from build123d import *

# Parameters (mm, degrees)
F0_W     = 60.325
F0_H     = 104.775
F1_DEPTH = 66.675
F3_DEPTH = 34.925
F5_DEPTH = 22.225
F6_W     = 26.9875
F6_H     = 6.35
F6_W_2   = 25.4
F7_DEPTH = 60.326
F9_DEPTH = 60.326


with BuildPart() as f1:
    # F0 (on Top) → F1 (new body)
    with BuildSketch(Plane.XY):
        Rectangle(F0_W, F0_H)
    extrude(amount=F1_DEPTH)

    # F2 (on face) → F3 (cut)
    with BuildSketch(Plane.YZ.offset(30.1625)):
        Polygon((-52.3875, 34.8233953258), (-52.3875, 15.875), (52.3875, 41.275), (52.3875, 60.2233953258), align=None)
    extrude(amount=-F3_DEPTH, mode=Mode.SUBTRACT)

    # F4 (on face) → F5 (cut)
    with BuildSketch(Plane.YZ.offset(30.1625)):
        Polygon((7.9375, 0), (7.9375, 30.4992424242), (-26.9875, 22.0325757576), (-26.9875, 0), align=None)
    extrude(amount=-F5_DEPTH, mode=Mode.SUBTRACT)

    # F6 (on face) → F7 (cut, through all)
    with BuildSketch(Plane.YZ.offset(30.1625)):
        with Locations((-13.49375, 3.175)):
            Rectangle(F6_W, F6_H)
        with Locations((-39.6875, 3.175)):
            Rectangle(F6_W_2, F6_H)
        Polygon((52.8014078736, 0), (52.5065548718, 6.35), (20.6375, 6.35), (20.6375, 0), align=None)
    extrude(amount=-F7_DEPTH, mode=Mode.SUBTRACT)

    # F8 (on face) → F9 (cut, through all)
    with BuildSketch(Plane.YZ.offset(30.1625)):
        Polygon((-7.9375, 45.5991529015), (-7.9375, 66.675), (-52.3875, 66.675), (-52.3875, 34.8233953258), align=None)
    extrude(amount=-F9_DEPTH, mode=Mode.SUBTRACT)


solid = f1.part
Can you work these out from the model? Positions are in its coordinate system, mm. A direction names the side the tool comes from. Coordinates: 2 decimals unless noted, no trailing zeros. Loops run counter-clockwise (first coordinate to the right, second up) from the corner with the lowest first, then second, coordinate; pieces in that order, holes last. Notation, with made-up numbers: M 1.5,28.5 L 7.5,28.5 A24 cw 7.5,39.5 Z; hole C -30,86 d4. An arc over 180 degrees is marked long. Return JSON: item names as keys, results as strings. Group by question number.
Item 1: Imagine slicing it at A-A (x = 22.5). Give the number of separate pieces and of enclosed holes in the cut face, and give its area (3 significant figures).
Item 2: On a 3-axis mill with a long thin cutter (end or side, diameter ignored), from which of +Z, -Z, +X, -X, +Y, -Y can I reach the whole of each face in a straight line? I mean faces 5 (the flat face through (0, 20.638, 3)), 6 (the flat face through (-6, -26, 6.35)), 7 (the flat face through (19, -26.988, 14)), 8 (the flat face through (7.938, -6, 15)). Say none if no direction works.
Item 3: I'm going to push flat-ended pins straight in: pin 1 Ø1.9 at (x, z) = (-19.5, 2.5) entering from -Y; pin 2 Ø3 at (x, z) = (5.5, 2) entering from +Y; pin 3 Ø1 at (x, z) = (-1.5, 56.5) entering from -Y; pin 4 Ø5 at (x, y) = (12, -22.5) entering from -Z. Where does each tip first touch, or does it pass through?
Item 4: Imagine slicing it at C-C (z = 13.5). Please give me the cut outline in (x, y).
Item 5: If I drill on L1, parallel to Z at x = -14, y = 29 (3 decimals); L2, parallel to Z at x = -4, y = 48 (3 decimals); L3, parallel to Y at x = -13, z = 3, over which ranges is the centre line in solid material (lowest first)? Write a range as from..to.
Item 6: Thinking about a two-plate mould opening in Z: for faces 1 (the flat face through (0, 10, 0)), 2 (the flat face through (30.162, 15, 58)), 3 (the flat face through (12.944, 22.647, 53.014)), 4 (the flat face through (-4.762, -1, 38)), which applies, released by +Z, released by -Z, zero draft, split by the parting line, or undercut?
Verdict:
{
 "1": {"separate pieces": "3", "enclosed holes": "0", "area": "2,540 mm^2"},
 "2": {"face 5": "-Z, +X, -X, +Y", "face 6": "-Z, +X, -X, -Y", "face 7": "+Z, -Z, +X", "face 8": "-Z, +X"},
 "3": {"pin 1": "stops at y = 0", "pin 2": "stops at y = 20.64", "pin 3": "stops at y = -7.94", "pin 4": "passes through"},
 "4": {"outline": "M -30.16,-52.39 L 30.16,-52.39 L 30.16,-26.99 L 7.94,-26.99 L 7.94,7.94 L 30.16,7.94 L 30.16,52.39 L -30.16,52.39 Z"},
 "5": {"L1": "z = 6.35..66.675", "L2": "z = 6.35..40.211, 59.16..66.675", "L3": "y = 0..20.64"},
 "6": {"face 1": "released by -Z", "face 2": "zero draft", "face 3": "undercut", "face 4": "undercut"}
}
